Geometry: final body of the model. Coordinates: model frame, mm. Round coordinates to 2 decimals unless told otherwise and drop trailing zeros. Loops run counter-clockwise (first coordinate to the right, second up) from the corner with the lowest first, then second, coordinate; pieces in that order, holes last. Notation, with made-up numbers: (11, -31) -> (47, -31) arc R15 cw to (47, -18) -> close; hole circle Ø5 at (-33.75, 83). An arc over 180 degrees is marked (long way). Answer in a Markdown table with one row per item.
```python
from build123d import *

# Parameters (mm, degrees)
SKETCH_3_W           = 44
SKETCH_3_H           = 24
EXTRUDE_2_DEPTH      = 1.5
SKETCH_4_R           = 1.05
CUT_EXTRUDE_1_DEPTH  = 1.5
SKETCH_5_R           = 1.1
CUT_EXTRUDE_2_DEPTH  = 1.5
SKETCH_6_R           = 1.15
CUT_EXTRUDE_3_DEPTH  = 1.5
SKETCH_7_R           = 1.2
CUT_EXTRUDE_4_DEPTH  = 1.5
SKETCH_8_R           = 1.25
CUT_EXTRUDE_6_DEPTH  = 1.5
SKETCH_10_R          = 1.3
CUT_EXTRUDE_7_DEPTH  = 1.5
SKETCH_11_R          = 1.35
CUT_EXTRUDE_8_DEPTH  = 1.5
SKETCH_12_R          = 1.4
CUT_EXTRUDE_9_DEPTH  = 1.5
SKETCH_13_R          = 1.45
CUT_EXTRUDE_10_DEPTH = 1.5
SKETCH_14_R          = 1.5
CUT_EXTRUDE_11_DEPTH = 1.5


with BuildPart() as part:
    # 草图3 → 凸台-拉伸2 (new body)
    with BuildSketch(Plane.XY):
        with Locations((22, 12)):
            Rectangle(SKETCH_3_W, SKETCH_3_H)
    extrude(amount=EXTRUDE_2_DEPTH)

    # 草图4 → 切除-拉伸1 (cut)
    with BuildSketch(Plane.XY):
        with Locations((4, 4)):
            Circle(SKETCH_4_R)
        with Locations((4, 8)):
            Circle(SKETCH_4_R)
        with Locations((4, 12)):
            Circle(SKETCH_4_R)
        with Locations((4, 16)):
            Circle(SKETCH_4_R)
        with Locations((4, 20)):
            Circle(SKETCH_4_R)
    extrude(amount=CUT_EXTRUDE_1_DEPTH, mode=Mode.SUBTRACT)

    # 草图5 → 切除-拉伸2 (cut)
    with BuildSketch(Plane.XY):
        with Locations((8, 4)):
            Circle(SKETCH_5_R)
        with Locations((8, 8)):
            Circle(SKETCH_5_R)
        with Locations((8, 12)):
            Circle(SKETCH_5_R)
        with Locations((8, 16)):
            Circle(SKETCH_5_R)
        with Locations((8, 20)):
            Circle(SKETCH_5_R)
    extrude(amount=CUT_EXTRUDE_2_DEPTH, mode=Mode.SUBTRACT)

    # 草图6 → 切除-拉伸3 (cut)
    with BuildSketch(Plane.XY):
        with Locations((12, 4)):
            Circle(SKETCH_6_R)
        with Locations((12, 8)):
            Circle(SKETCH_6_R)
        with Locations((12, 12)):
            Circle(SKETCH_6_R)
        with Locations((12, 16)):
            Circle(SKETCH_6_R)
        with Locations((12, 20)):
            Circle(SKETCH_6_R)
    extrude(amount=CUT_EXTRUDE_3_DEPTH, mode=Mode.SUBTRACT)

    # 草图7 → 切除-拉伸4 (cut)
    with BuildSketch(Plane.XY):
        with Locations((16, 4)):
            Circle(SKETCH_7_R)
        with Locations((16, 8)):
            Circle(SKETCH_7_R)
        with Locations((16, 12)):
            Circle(SKETCH_7_R)
        with Locations((16, 16)):
            Circle(SKETCH_7_R)
        with Locations((16, 20)):
            Circle(SKETCH_7_R)
    extrude(amount=CUT_EXTRUDE_4_DEPTH, mode=Mode.SUBTRACT)

    # 草图8 → 切除-拉伸6 (cut)
    with BuildSketch(Plane.XY):
        with Locations((20, 4)):
            Circle(SKETCH_8_R)
        with Locations((20, 8)):
            Circle(SKETCH_8_R)
        with Locations((20, 12)):
            Circle(SKETCH_8_R)
        with Locations((20, 16)):
            Circle(SKETCH_8_R)
        with Locations((20, 20)):
            Circle(SKETCH_8_R)
    extrude(amount=CUT_EXTRUDE_6_DEPTH, mode=Mode.SUBTRACT)

    # 草图10 → 切除-拉伸7 (cut)
    with BuildSketch(Plane.XY):
        with Locations((24, 4)):
            Circle(SKETCH_10_R)
        with Locations((24, 8)):
            Circle(SKETCH_10_R)
        with Locations((24, 12)):
            Circle(SKETCH_10_R)
        with Locations((24, 16)):
            Circle(SKETCH_10_R)
        with Locations((24, 20)):
            Circle(SKETCH_10_R)
    extrude(amount=CUT_EXTRUDE_7_DEPTH, mode=Mode.SUBTRACT)

    # 草图11 → 切除-拉伸8 (cut)
    with BuildSketch(Plane.XY):
        with Locations((28, 4)):
            Circle(SKETCH_11_R)
        with Locations((28, 8)):
            Circle(SKETCH_11_R)
        with Locations((28, 12)):
            Circle(SKETCH_11_R)
        with Locations((28, 16)):
            Circle(SKETCH_11_R)
        with Locations((28, 20)):
            Circle(SKETCH_11_R)
    extrude(amount=CUT_EXTRUDE_8_DEPTH, mode=Mode.SUBTRACT)

    # 草图12 → 切除-拉伸9 (cut)
    with BuildSketch(Plane.XY):
        with Locations((32, 4)):
            Circle(SKETCH_12_R)
        with Locations((32, 8)):
            Circle(SKETCH_12_R)
        with Locations((32, 12)):
            Circle(SKETCH_12_R)
        with Locations((32, 16)):
            Circle(SKETCH_12_R)
        with Locations((32, 20)):
            Circle(SKETCH_12_R)
    extrude(amount=CUT_EXTRUDE_9_DEPTH, mode=Mode.SUBTRACT)

    # 草图13 → 切除-拉伸10 (cut)
    with BuildSketch(Plane.XY):
        with Locations((36, 4)):
            Circle(SKETCH_13_R)
        with Locations((36, 8)):
            Circle(SKETCH_13_R)
        with Locations((36, 12)):
            Circle(SKETCH_13_R)
        with Locations((36, 16)):
            Circle(SKETCH_13_R)
        with Locations((36, 20)):
            Circle(SKETCH_13_R)
    extrude(amount=CUT_EXTRUDE_10_DEPTH, mode=Mode.SUBTRACT)

    # 草图14 → 切除-拉伸11 (cut)
    with BuildSketch(Plane.XY):
        with Locations((40, 4)):
            Circle(SKETCH_14_R)
        with Locations((40, 8)):
            Circle(SKETCH_14_R)
        with Locations((40, 12)):
            Circle(SKETCH_14_R)
        with Locations((40, 16)):
            Circle(SKETCH_14_R)
        with Locations((40, 20)):
            Circle(SKETCH_14_R)
    extrude(amount=CUT_EXTRUDE_11_DEPTH, mode=Mode.SUBTRACT)


solid = part.part
```
Item 1: First-contact query: P1, Ø1.5, axis at x = 8, y = 16, coming from the +Z side. Flat tip, straight axial feed; report the tip coordinate or a pass-through.
Ans:
| item | result |
|---|---|
| P1 | through |
Item 2: Section query A-A, the plane x = 32. Output: boundary loops of the cut face in (y, z), and give its area (3 significant figures).
Ans:
| item | result |
|---|---|
| outline | (0, 0) -> (2.6, 0) -> (2.6, 1.5) -> (0, 1.5) -> close; (5.4, 0) -> (6.6, 0) -> (6.6, 1.5) -> (5.4, 1.5) -> close; (9.4, 0) -> (10.6, 0) -> (10.6, 1.5) -> (9.4, 1.5) -> close; (13.4, 0) -> (14.6, 0) -> (14.6, 1.5) -> (13.4, 1.5) -> close; (17.4, 0) -> (18.6, 0) -> (18.6, 1.5) -> (17.4, 1.5) -> close; (21.4, 0) -> (24, 0) -> (24, 1.5) -> (21.4, 1.5) -> close |
| area | 15.0 mm2 |
Item 3: Section query C-C, the plane z = 0.4. State how many separate pieces and enclosed holes the cut face has, and give its area (3 significant figures).
Ans:
| item | result |
|---|---|
| separate pieces | 1 |
| enclosed holes | 50 |
| area | 797 mm2 |
Item 4: Ray query, L1, parallel to Y at x = 28, z = 0.9; L2, parallel to Y at x = 32, z = 0.45. Return the intervals inside material, ascending.
Ans:
| item | result |
|---|---|
| L1 | 0 to 2.65, 5.35 to 6.65, 9.35 to 10.65, 13.35 to 14.65, 17.35 to 18.65, 21.35 to 24 |
| L2 | 0 to 2.6, 5.4 to 6.6, 9.4 to 10.6, 13.4 to 14.6, 17.4 to 18.6, 21.4 to 24 |
Item 5: Mould query, pull axis Y, two halves, no side actions, for faces 1 (the cylindrical face through (20.672, 17.054, 0.74)), 2 (the flat face through (44, 12, 1)), 3 (the cylindrical face through (30.89, 19.15, 0.74)). Classes: released by +Y, released by -Y, zero draft, split by the parting line, or undercut.
Ans:
| item | result |
|---|---|
| face 1 | undercut |
| face 2 | zero draft |
| face 3 | undercut |
Item 6: Section query B-B, the plane x = 40. Output: boundary loops of the cut face in (y, z), and give its area (3 significant figures).
Ans:
| item | result |
|---|---|
| outline | (0, 0) -> (2.5, 0) -> (2.5, 1.5) -> (0, 1.5) -> close; (5.5, 0) -> (6.5, 0) -> (6.5, 1.5) -> (5.5, 1.5) -> close; (9.5, 0) -> (10.5, 0) -> (10.5, 1.5) -> (9.5, 1.5) -> close; (13.5, 0) -> (14.5, 0) -> (14.5, 1.5) -> (13.5, 1.5) -> close; (17.5, 0) -> (18.5, 0) -> (18.5, 1.5) -> (17.5, 1.5) -> close; (21.5, 0) -> (24, 0) -> (24, 1.5) -> (21.5, 1.5) -> close |
| area | 13.5 mm2 |
